Part model, mm, in its own coordinate system. Round coordinates to 2 decimals unless told otherwise and drop trailing zeros. Order: outer loops, then holes, each group sorted by start corner. A loop starts at its lowest first (then second) coordinate and runs counter-clockwise, first axis right, second up. Notation, with made-up numbers: (29.5, -31) - (52.5, -31) arc R30 ccw to (52.5, -8) - close; hole circle Ø5 at (75.5, 14). An arc over 180 degrees is marked (long way). Return JSON: item names as keys, results as strings. Group by question number.
Item 1: Saw through at D-D on y = 0.55. List the corners of the cut face in (x, z) (1 decimal), and give its area (3 significant figures).
Item 2: Saw through at C-C on z = 12.7. List the corners of the cut face in (x, y).
Item 3: Drop flat-ended pins along their axis: pin 1 (4 mm diameter, centred on x = -6, z = 10, fed in from -Y); pin 2 (0.8 mm diameter, centred on y = 0.5, z = -22, fed in from +X) (3 decimals); pin 3 (0.5 mm diameter, centred on x = 3.5, y = -0.5, fed in from +Z); pin 4 (5 mm diameter, centred on x = -12.5, z = 13.5, fed in from +Y). Give the stop position or say it passes through.
Item 4: Probe probe 1 along X at (y, z) = (-0.6, 9.5); probe 2 along X at (y, z) = (-0.2, -30) (3 decimals); probe 3 along X at (y, z) = (-0.5, 12.7). List the from-to ranges inside material, lowest first.
Item 5: Saw through at A-A on z = -2. List the corners of the cut face in (x, y), and give its area (3 significant figures).
Item 6: Saw through at B-B on x = 0. List the corners of the cut face in (y, z).
```python
from build123d import *

# Parameters (mm, degrees)
SKETCH1_W           = 6.35
SKETCH1_H           = 19.05
BOSS_EXTRUDE1_DEPTH = 0.79375
SKETCH2_W           = 6.35
SKETCH2_H           = 4.7625
CUT_EXTRUDE1_DEPTH  = 0.79375
SKETCH3_R           = 0.80645
SKETCH3_R_2         = 2.38125
SKETCH3_R_3         = 1.936420783
CUT_EXTRUDE2_DEPTH  = 1.5875


with BuildPart() as part:
    # Sketch1 → Boss-Extrude1 (new, symmetric)
    with BuildSketch(Plane(origin=(0, 0, 0), x_dir=(1, 0, 0), z_dir=(0, 1, 0))):
        Polygon((-3.175, 15.08125), (-14.2875, 15.08125), (-14.2875, -15.08125), (-7.9375, -15.08125), (-7.9375, 5.55625), (7.9375, 5.55625), (7.9375, -15.08125), (14.2875, -15.08125), (14.2875, 15.08125), (3.175, 15.08125), align=None)
        with Locations((0, 24.60625)):
            Rectangle(SKETCH1_W, SKETCH1_H)
    extrude(amount=BOSS_EXTRUDE1_DEPTH, both=True)

    # Sketch2 → Cut-Extrude1 (cut)
    with BuildSketch(Plane(origin=(0, 0.79375, 0), x_dir=(1, 0, 0), z_dir=(0, 1, 0))):
        with Locations((-11.1125, -12.7)):
            Rectangle(SKETCH2_W, SKETCH2_H)
        with Locations((11.1125, -12.7)):
            Rectangle(SKETCH2_W, SKETCH2_H)
    extrude(amount=-CUT_EXTRUDE1_DEPTH, mode=Mode.SUBTRACT)

    # Sketch3 → Cut-Extrude2 (cut)
    with BuildSketch(Plane(origin=(0, 0.79375, 0), x_dir=(1, 0, 0), z_dir=(0, 1, 0))):
        with Locations(Location((-11.1125, -12.7, 0), (0, 0, 270))):
            Circle(SKETCH3_R)
        with Locations(Location((-7.9375, 10.31875, 0), (0, 0, 270))):
            Circle(SKETCH3_R_2)
        with Locations(Location((11.1125, -12.7, 0), (0, 0, 270))):
            Circle(SKETCH3_R)
        with Locations(Location((7.9375, 10.31875, 0), (0, 0, 270))):
            Circle(SKETCH3_R_2)
        with Locations(Location((0, 18.44201602, 0), (0, 0, 270))):
            Circle(SKETCH3_R_3)
        with Locations(Location((0, 29.994029814, 0), (0, 0, 270))):
            Circle(SKETCH3_R_3)
    extrude(amount=-CUT_EXTRUDE2_DEPTH, mode=Mode.SUBTRACT)


solid = part.part
```
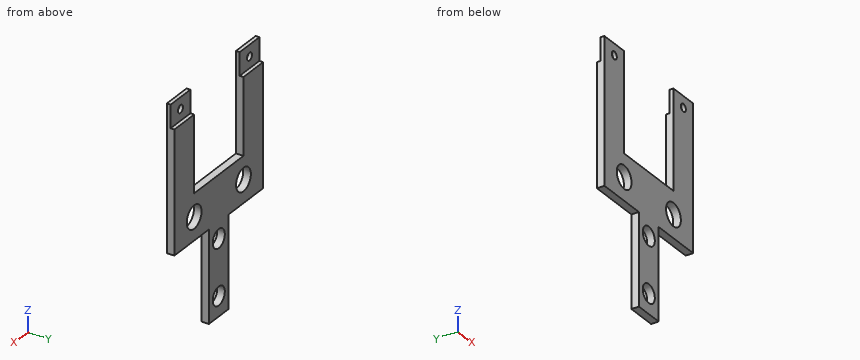
Filled in:
{
 "1": {"outline": "(-14.3, -15.1) - (-3.2, -15.1) - (-3.2, -34.1) - (3.2, -34.1) - (3.2, -15.1) - (14.3, -15.1) - (14.3, 10.3) - (7.9, 10.3) - (7.9, -5.6) - (-7.9, -5.6) - (-7.9, 10.3) - (-14.3, 10.3) - close; hole circle Ø4.8 at (-7.9, -10.3); hole circle Ø3.9 at (0, -30); hole circle Ø3.9 at (0, -18.4); hole circle Ø4.8 at (7.9, -10.3)", "area": "536 mm^2"},
 "2": {"outline": "(-14.29, -0.79) - (-11.92, -0.79) - (-11.92, 0) - (-14.29, 0) - close; (-10.31, -0.79) - (-7.94, -0.79) - (-7.94, 0) - (-10.31, 0) - close; (7.94, -0.79) - (10.31, -0.79) - (10.31, 0) - (7.94, 0) - close; (11.92, -0.79) - (14.29, -0.79) - (14.29, 0) - (11.92, 0) - close"},
 "3": {"pin 1": "stops at y = -0.79", "pin 2": "stops at x = 3.175", "pin 3": "stops at z = -5.56", "pin 4": "stops at y = 0"},
 "4": {"probe 1": "x = -14.29 to -7.94, 7.94 to 14.29", "probe 2": "x = -3.175 to -1.936, 1.936 to 3.175", "probe 3": "x = -14.29 to -11.92, -10.31 to -7.94, 7.94 to 10.31, 11.92 to 14.29"},
 "5": {"outline": "(-14.29, -0.79) - (-7.94, -0.79) - (-7.94, 0.79) - (-14.29, 0.79) - close; (7.94, -0.79) - (14.29, -0.79) - (14.29, 0.79) - (7.94, 0.79) - close", "area": "20.2 mm^2"},
 "6": {"outline": "(-0.79, -34.13) - (0.79, -34.13) - (0.79, -31.93) - (-0.79, -31.93) - close; (-0.79, -28.06) - (0.79, -28.06) - (0.79, -20.38) - (-0.79, -20.38) - close; (-0.79, -16.51) - (0.79, -16.51) - (0.79, -5.56) - (-0.79, -5.56) - close"}
}
